Autodesk Inventor part; units mm, degrees
ref_plane "YZ Plane" through (0, 0, 0) normal (1, 0, 0) x (0, 1, 0)
ref_plane "XZ Plane" through (0, 0, 0) normal (0, 1, 0) x (-1, 0, 0)
ref_plane "XY Plane" through (0, 0, 0) normal (0, 0, 1) x (1, 0, 0)
sketch "Sketch1" plane through (0, 0, 0) normal (0, 0, 1) x (1, 0, 0)
  circle A0 centre (0, 0) radius 15
  circle A1 centre (0, 0) radius 3.6
  dimension "d0" = 30
  dimension "d1" = 7.2
extrude "Extrusion1" add sketch "Sketch1" along normal blind 10
sketch "Sketch3" plane through (0, 0, 10) normal (0, 0, 1) x (1, 0, 0)
  line L0 (0, 0) -> (25, 0) construction
  arc A0 (18.8792, 0.8) -> (14.8792, 1.9) centre (12.94, -12.9741) ccw
  circle A1 centre (0, 0) radius 15
  arc A2 (18.8792, -0.8) -> (18.8792, 0.8) centre (-1.1048, 0) ccw
  arc A3 (14.8792, -1.9) -> (18.8792, -0.8) centre (12.94, 12.9741) ccw
  arc A4 (14.8792, -1.9) -> (14.8792, 1.9) centre (0, 0) ccw
  arc A5 (17.467, 7.2088) -> (13.332, 6.8744) centre (16.5971, -7.7659) ccw
  arc A6 (18.0142, 5.7053) -> (17.467, 7.2088) centre (-1.0382, -0.3779) ccw
  arc A7 (14.6317, 3.3036) -> (18.0142, 5.7053) centre (7.7223, 16.6175) ccw
  arc A8 (14.6317, 3.3036) -> (13.332, 6.8744) centre (0, 0) ccw
  arc A9 (13.9481, 12.7481) -> (10.1768, 11.0196) centre (18.2523, -1.6211) ccw
  arc A10 (14.9765, 11.5225) -> (13.9481, 12.7481) centre (-0.8463, -0.7102) ccw
  arc A11 (12.6194, 8.1087) -> (14.9765, 11.5225) centre (1.573, 18.2565) ccw
  arc A12 (12.6194, 8.1087) -> (10.1768, 11.0196) centre (0, 0) ccw
  arc A13 (8.7468, 16.7498) -> (5.7941, 13.8357) centre (17.7059, 4.7193) ccw
  arc A14 (10.1324, 15.9498) -> (8.7468, 16.7498) centre (-0.5524, -0.9568) ccw
  arc A15 (9.085, 11.9357) -> (10.1324, 15.9498) centre (-4.7659, 17.6935) ccw
  arc A16 (9.085, 11.9357) -> (5.7941, 13.8357) centre (0, 0) ccw
  arc A17 (2.4905, 18.7313) -> (0.7126, 14.9831) centre (15.024, 10.4905) ccw
  arc A18 (4.0662, 18.4534) -> (2.4905, 18.7313) centre (-0.1918, -1.088) ccw
  arc A19 (4.4549, 14.3232) -> (4.0662, 18.4534) centre (-10.53, 14.9964) ccw
  arc A20 (4.4549, 14.3232) -> (0.7126, 14.9831) centre (0, 0) ccw
  arc A21 (-4.0662, 18.4534) -> (-4.4549, 14.3232) centre (10.53, 14.9964) ccw
  arc A22 (-2.4905, 18.7313) -> (-4.0662, 18.4534) centre (0.1918, -1.088) ccw
  arc A23 (-0.7126, 14.9831) -> (-2.4905, 18.7313) centre (-15.024, 10.4905) ccw
  arc A24 (-0.7126, 14.9831) -> (-4.4549, 14.3232) centre (0, 0) ccw
  arc A25 (-10.1324, 15.9498) -> (-9.085, 11.9357) centre (4.7659, 17.6935) ccw
  arc A26 (-8.7468, 16.7498) -> (-10.1324, 15.9498) centre (0.5524, -0.9568) ccw
  arc A27 (-5.7941, 13.8357) -> (-8.7468, 16.7498) centre (-17.7059, 4.7193) ccw
  arc A28 (-5.7941, 13.8357) -> (-9.085, 11.9357) centre (0, 0) ccw
  arc A29 (-14.9765, 11.5225) -> (-12.6194, 8.1087) centre (-1.573, 18.2565) ccw
  arc A30 (-13.9481, 12.7481) -> (-14.9765, 11.5225) centre (0.8463, -0.7102) ccw
  arc A31 (-10.1768, 11.0196) -> (-13.9481, 12.7481) centre (-18.2523, -1.6211) ccw
  arc A32 (-10.1768, 11.0196) -> (-12.6194, 8.1087) centre (0, 0) ccw
  arc A33 (-18.0142, 5.7053) -> (-14.6317, 3.3036) centre (-7.7223, 16.6175) ccw
  arc A34 (-17.467, 7.2088) -> (-18.0142, 5.7053) centre (1.0382, -0.3779) ccw
  arc A35 (-13.332, 6.8744) -> (-17.467, 7.2088) centre (-16.5971, -7.7659) ccw
  arc A36 (-13.332, 6.8744) -> (-14.6317, 3.3036) centre (0, 0) ccw
  arc A37 (-18.8792, -0.8) -> (-14.8792, -1.9) centre (-12.94, 12.9741) ccw
  arc A38 (-18.8792, 0.8) -> (-18.8792, -0.8) centre (1.1048, 0) ccw
  arc A39 (-14.8792, 1.9) -> (-18.8792, 0.8) centre (-12.94, -12.9741) ccw
  arc A40 (-14.8792, 1.9) -> (-14.8792, -1.9) centre (0, 0) ccw
  arc A41 (-17.467, -7.2088) -> (-13.332, -6.8744) centre (-16.5971, 7.7659) ccw
  arc A42 (-18.0142, -5.7053) -> (-17.467, -7.2088) centre (1.0382, 0.3779) ccw
  arc A43 (-14.6317, -3.3036) -> (-18.0142, -5.7053) centre (-7.7223, -16.6175) ccw
  arc A44 (-14.6317, -3.3036) -> (-13.332, -6.8744) centre (0, 0) ccw
  arc A45 (-13.9481, -12.7481) -> (-10.1768, -11.0196) centre (-18.2523, 1.6211) ccw
  arc A46 (-14.9765, -11.5225) -> (-13.9481, -12.7481) centre (0.8463, 0.7102) ccw
  arc A47 (-12.6194, -8.1087) -> (-14.9765, -11.5225) centre (-1.573, -18.2565) ccw
  arc A48 (-12.6194, -8.1087) -> (-10.1768, -11.0196) centre (0, 0) ccw
  arc A49 (-8.7468, -16.7498) -> (-5.7941, -13.8357) centre (-17.7059, -4.7193) ccw
  arc A50 (-10.1324, -15.9498) -> (-8.7468, -16.7498) centre (0.5524, 0.9568) ccw
  arc A51 (-9.085, -11.9357) -> (-10.1324, -15.9498) centre (4.7659, -17.6935) ccw
  arc A52 (-9.085, -11.9357) -> (-5.7941, -13.8357) centre (0, 0) ccw
  arc A53 (-2.4905, -18.7313) -> (-0.7126, -14.9831) centre (-15.024, -10.4905) ccw
  arc A54 (-4.0662, -18.4534) -> (-2.4905, -18.7313) centre (0.1918, 1.088) ccw
  arc A55 (-4.4549, -14.3232) -> (-4.0662, -18.4534) centre (10.53, -14.9964) ccw
  arc A56 (-4.4549, -14.3232) -> (-0.7126, -14.9831) centre (0, 0) ccw
  arc A57 (4.0662, -18.4534) -> (4.4549, -14.3232) centre (-10.53, -14.9964) ccw
  arc A58 (2.4905, -18.7313) -> (4.0662, -18.4534) centre (-0.1918, 1.088) ccw
  arc A59 (0.7126, -14.9831) -> (2.4905, -18.7313) centre (15.024, -10.4905) ccw
  arc A60 (0.7126, -14.9831) -> (4.4549, -14.3232) centre (0, 0) ccw
  arc A61 (10.1324, -15.9498) -> (9.085, -11.9357) centre (-4.7659, -17.6935) ccw
  arc A62 (8.7468, -16.7498) -> (10.1324, -15.9498) centre (-0.5524, 0.9568) ccw
  arc A63 (5.7941, -13.8357) -> (8.7468, -16.7498) centre (17.7059, -4.7193) ccw
  arc A64 (5.7941, -13.8357) -> (9.085, -11.9357) centre (0, 0) ccw
  arc A65 (14.9765, -11.5225) -> (12.6194, -8.1087) centre (1.573, -18.2565) ccw
  arc A66 (13.9481, -12.7481) -> (14.9765, -11.5225) centre (-0.8463, 0.7102) ccw
  arc A67 (10.1768, -11.0196) -> (13.9481, -12.7481) centre (18.2523, 1.6211) ccw
  arc A68 (10.1768, -11.0196) -> (12.6194, -8.1087) centre (0, 0) ccw
  arc A69 (18.0142, -5.7053) -> (14.6317, -3.3036) centre (7.7223, -16.6175) ccw
  arc A70 (17.467, -7.2088) -> (18.0142, -5.7053) centre (-1.0382, 0.3779) ccw
  arc A71 (13.332, -6.8744) -> (17.467, -7.2088) centre (16.5971, 7.7659) ccw
  arc A72 (13.332, -6.8744) -> (14.6317, -3.3036) centre (0, 0) ccw
  point P0 (18.8952, 0)
  point P1 (17.7557, 6.4625)
  point P2 (14.4746, 12.1456)
  point P3 (9.4476, 16.3637)
  point P4 (3.2811, 18.6081)
  point P5 (-3.2811, 18.6081)
  point P6 (-9.4476, 16.3637)
  point P7 (-14.4746, 12.1456)
  point P8 (-17.7557, 6.4625)
  point P9 (-18.8952, 0)
  point P10 (-17.7557, -6.4625)
  point P11 (-14.4746, -12.1456)
  point P12 (-9.4476, -16.3637)
  point P13 (-3.2811, -18.6081)
  point P14 (3.2811, -18.6081)
  point P15 (9.4476, -16.3637)
  point P16 (14.4746, -12.1456)
  point P17 (17.7557, -6.4625)
  dimension "d8" = 25
  dimension "d9" = 15
  dimension "d10" = 1.6
  dimension "d11" = 20
  dimension "d12" = 4
  dimension "d13" = 1.1
  dimension "d14" = 15
  dimension "d15" = 1.1
  dimension "d16" = 4
  dimension "d19" = 360
extrude "Extrusion3" add sketch "Sketch3" against normal blind 10 contours A2 A3 A1 A0 | A1 A5 A6 A7 | A69 A70 A71 A1 | A1 A9 A10 A11 | A65 A66 A67 A1 | A1 A13 A14 A15 | A61 A62 A63 A1 | A1 A17 A18 A19 | A57 A58 A59 A1 | A1 A21 A22 A23 | A53 A54 A55 A1 | A1 A25 A26 A27 | A49 A50 A51 A1 | A1 A29 A30 A31 | A45 A46 A47 A1 | A1 A33 A34 A35 | A41 A42 A43 A1 | A1 A37 A38 A39
sketch "Sketch2" plane through (0, 0, 10) normal (0, 0, 1) x (1, 0, 0)
  circle A0 centre (9.1587, 1.6149) radius 1.5
  circle A1 centre (0, 0) radius 15 construction
  circle A2 centre (0, 0) radius 3.6 construction
  circle A3 centre (0, 0) radius 3.6 construction
  circle A4 centre (0, 0) radius 15 construction
  arc A5 (14.8792, 1.9) -> (14.6317, 3.3036) centre (0, 0) ccw
  line L0 (3.5453, 0.6251) -> (14.7721, 2.6047) construction
  line L1 (0, 0) -> (3.5453, 0.6251) construction
  line L2 (0, 0) -> (14.7721, 2.6047) construction
  dimension "d4" = 3
extrude "Extrusion2" cut sketch "Sketch2" against normal through all
properties part number "GA002" material "ABS Plastic"
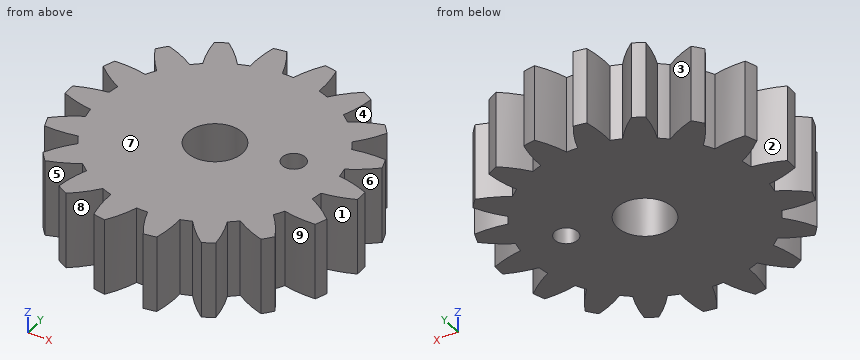
Part model, mm, in its own coordinate system. Face numbers are marked on the shaded views. A direction names the side the tool comes from. Give positions to 0.01 mm unless a question says otherwise; leave off trailing zeros. Loops run counter-clockwise (first coordinate to the right, second up) from the corner with the lowest first, then second, coordinate; pieces in that order, holes last. Notation, with made-up numbers: M 52,65 L 104,65 A19 cw 104,88 Z; hole C 71.25,10 d7. An arc over 180 degrees is marked long. Return JSON: item names as keys, results as strings.
1) Saw through at A-A, the plane x = 0. List the corners of the cut face in (y, z).
Calculated:
{"outline": "M -15,0 L -3.6,0 L -3.6,10 L -15,10 Z; M 3.6,0 L 15,0 L 15,10 L 3.6,10 Z"}
2) Pull direction X, two halves, no side cores. Call the marked faces 6, 7, 8 and 9: released by +X, released by -X, zero draft, split by the parting line, or undercut.
Calculated:
{"face 6": "released by +X", "face 7": "zero draft", "face 8": "undercut", "face 9": "undercut"}
3) 3-axis set-ups, long thin cutter, end or side, ignore diameter. For the marked faces 1, 2, 3, 4 and 5: which of +Z, -Z, +X, -X, +Y, -Y reach the whole face in a straight line?
Calculated:
{"face 1": "+Z, -Z, +X", "face 2": "+Z, -Z, -X", "face 3": "+Z, -Z, +Y", "face 4": "+Z, -Z", "face 5": "+Z, -Z, -Y"}
4) Saw through at C-C, the plane y = 9.5. List the corners of the cut face in (x, z).
Calculated:
{"outline": "M -13.75,0 L 13.75,0 L 13.75,10 L -13.75,10 Z"}
5) Drill centre lines: line 1 (Y direction, x = 16, z = 9.25); line 2 (X direction, y = 12, z = 7); line 3 (X direction, y = -16.5, z = 7). Where is each one in solid material? Low to high.
Calculated:
{"line 1": "y = -7.22 to -4.11, -1.71 to 1.71, 4.11 to 7.22", "line 2": "x = -14.6 to -11.97, -9.11 to 9.11, 11.97 to 14.6", "line 3": "x = -9.21 to -8.42, -4.39 to -1.28, 1.28 to 4.39, 8.42 to 9.21"}
6) Saw through at D-D, the plane z = 9. Count the separate pieces of the cut face and the enclosed holes in it, then the cut area to 3 significant figures.
Calculated:
{"separate pieces": "1", "enclosed holes": "2", "area": "863 mm2"}
7) Saw through at B-B, the plane x = 16.5. List the corners of the cut face in (y, z), then the cut area to 3 significant figures.
Calculated:
{"outline": "M -7.23,0 L -4.45,0 L -4.45,10 L -7.23,10 Z; M -1.6,0 L 1.6,0 L 1.6,10 L -1.6,10 Z; M 4.45,0 L 7.23,0 L 7.23,10 L 4.45,10 Z", "area": "87.5 mm2"}
8) Flat gauge pins, fed straight in: pin 1 Ø2.5 at (x, y) = (9.16, 1.61) entering from -Z; pin 2 Ø2 at (x, z) = (-6, 7) entering from +Y; pin 3 Ø3 at (x, z) = (12.5, 1) entering from +Y; pin 4 Ø1.5 at (y, z) = (-1.5, 4) entering from +X. Where does each tip first touch, or does it go through?
Calculated:
{"pin 1": "passes through", "pin 2": "stops at y = 15.23", "pin 3": "stops at y = 12.75", "pin 4": "stops at x = 18.88"}
